Could you check a few things on this drawing? It's one solid part, dimensions in mm from its lowest x, y, z. A direction names the side the tool comes from. Coordinates: 2 decimals unless noted, no trailing zeros. Order: outer loops, then holes, each group sorted by start corner. A loop starts at its lowest first (then second) coordinate and runs counter-clockwise, first axis right, second up.
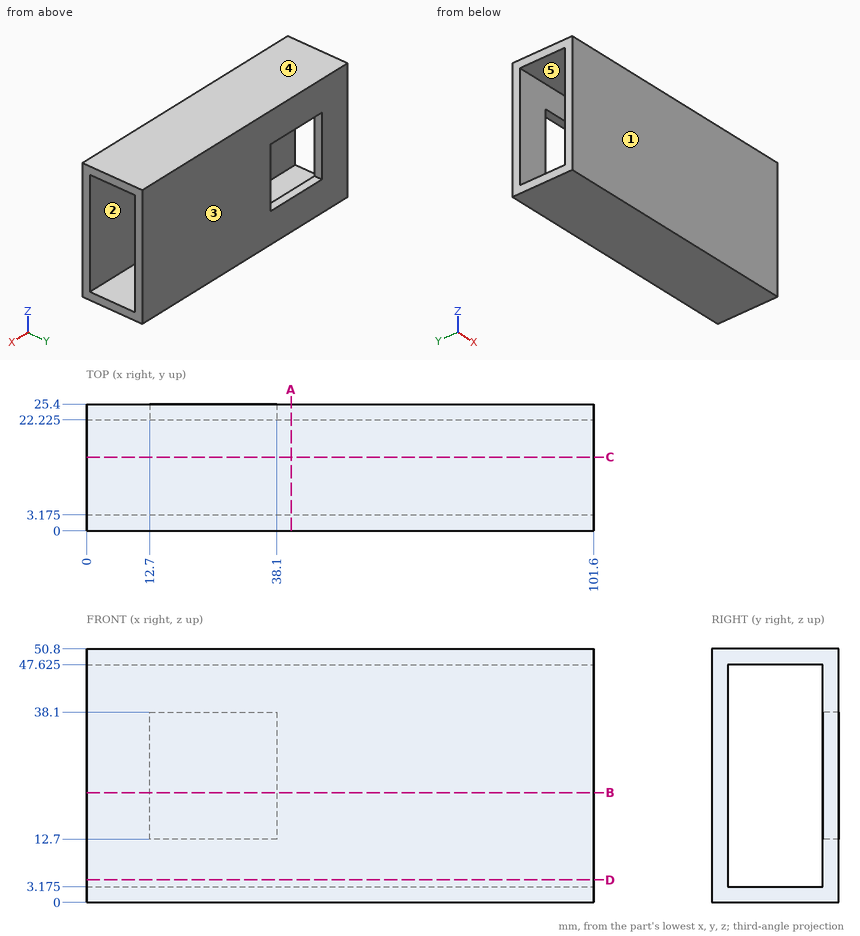
Q1. If we section it at C-C on y = 14.75: Write out the boundary of the cut face in (x, z) (3 decimals).
Q2. If we section it at D-D on z = 4.5: Write out the boundary of the cut face in (x, y) (3 decimals), then the cut area to 3 significant figures.
Q3. If we section it at A-A on x = 41: Write out the boundary of the cut face in (y, z) (3 decimals).
Q4. I need wall thicknesses on L1, parallel to Y at x = 84, z = 30 (3 decimals); L2, parallel to Z at x = 33, y = 15 (3 decimals). Which ranges of each line are inside material? Lowest first, please.
Q5. Will this pin go through, and if not, where does the flat tip stop? pin 1 (12 mm diameter, centred on y = 12, z = 31.5, fed in from +X).
Q6. If we section it at B-B on z = 22: Write out the boundary of the cut face in (x, y) (3 decimals).
Q7. For the marked faces 1 and 2, which set-ups out of +Z, -Z, +X, -X, +Y, -Y let a thin tool reach every point of the face, with its end or its side?
Q8. We'd pull the mould along Y, two halves only. Please class the marked faces 3, 4 and 5: pulls with the +Y half, pulls with the -Y half, needs draft (parallel to the pull), parting line crosses it, or undercut.
Reply:
1. outline: (0, 0) - (101.6, 0) - (101.6, 3.175) - (0, 3.175) - close; (0, 47.625) - (101.6, 47.625) - (101.6, 50.8) - (0, 50.8) - close
2. outline: (0, 0) - (101.6, 0) - (101.6, 3.175) - (0, 3.175) - close; (0, 22.225) - (101.6, 22.225) - (101.6, 25.4) - (0, 25.4) - close
2. area: 645 mm2
3. outline: (0, 0) - (25.4, 0) - (25.4, 50.8) - (0, 50.8) - close; hole (3.175, 3.175) - (22.225, 3.175) - (22.225, 47.625) - (3.175, 47.625) - close
4. L1: y = 0 to 3.175, 22.225 to 25.4
4. L2: z = 0 to 3.175, 47.625 to 50.8
5. pin 1: passes through
6. outline: (0, 0) - (101.6, 0) - (101.6, 3.175) - (0, 3.175) - close; (0, 22.225) - (12.7, 22.225) - (12.7, 25.4) - (0, 25.4) - close; (38.1, 22.225) - (101.6, 22.225) - (101.6, 25.4) - (38.1, 25.4) - close
7. face 1: +Z, -Z, +X, -X, -Y
7. face 2: +X, -X
8. face 3: pulls with the +Y half
8. face 4: needs draft
8. face 5: undercut
